```python
from build123d import *

# Parameters (mm, degrees)
BOSS_EXTRUDE1_DEPTH = 609.6
CUT_EXTRUDE1_DEPTH  = 38.1


with BuildPart() as part:
    # Sketch1 → Boss-Extrude1 (new body)
    with BuildSketch(Plane(origin=(0, 0, 0), x_dir=(1, 0, 0), z_dir=(0, 1, 0))):
        Polygon((13.746380944, 0), (9.720159182, 9.720159182), (0, 13.746380944), (-9.720159182, 9.720159182), (-13.746380944, 0), (-9.720159182, -9.720159182), (0, -13.746380944), (9.720159182, -9.720159182), align=None)
    extrude(amount=BOSS_EXTRUDE1_DEPTH)

    # Sketch2 → Cut-Extrude1 (cut)
    with BuildSketch(Plane(origin=(0, 609.6, 0), x_dir=(1, 0, 0), z_dir=(0, 1, 0))):
        Polygon((-1.00655544, -14.163309858), (-10.726714622, 9.303230267), (1.00655544, 14.163309858), (10.726714622, -9.303230267), align=None)
    extrude(amount=-CUT_EXTRUDE1_DEPTH, mode=Mode.SUBTRACT)


solid = part.part
```
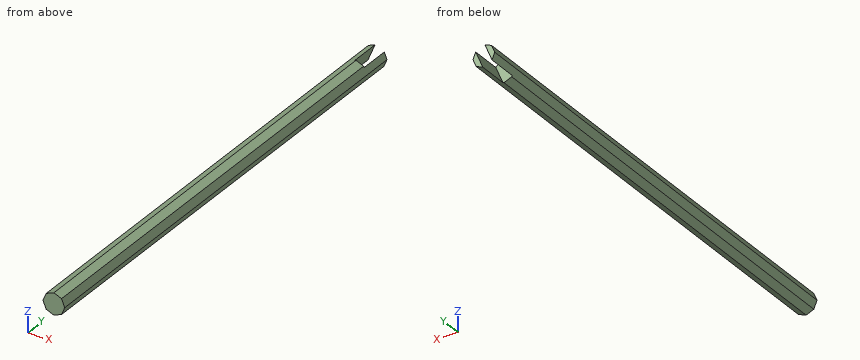
Read the model definition and answer for the solid it produces. Units are mm, in the model's axes. Give positions to 0.01 mm unless a question says otherwise; leave off trailing zeros. Write each loop counter-clockwise with the first axis right and the second up, starting at its lowest first coordinate (ties: lowest second). Pieces come first, ordered by that corner, then holes. Notation, with made-up numbers: (83, 79.25) - (91, 79.25) arc R9 cw to (91, 92.25) - close; hole circle Ø6 at (84.5, -12.75). An arc over 180 degrees is marked (long way). Write item = value, one per line. Start each with the question number.
Item 1: Each of these flat-tipped pins is pushed along its axis until it touches: P1, Ø4, axis at x = 7.5, y = 325.5, coming from the +Z side; P2, Ø1.5, axis at y = 313, z = -2, coming from the -X side; P3, Ø4, axis at y = 378.5, z = 7, coming from the +X side. Where does it stop, or does it pass through?
Item 2: Find the intervals of material crossed by probe 1 along X at (y, z) = (34.5, 9.5); probe 2 along Y at (x, z) = (4, 12); probe 3 along Z at (x, y) = (8.25, 161), in increasing order. Write a range as [from, to].
Item 3: Find section A-A (y = 50). Give the vertices of the cut face in (x, z).
Response:
q1.P1 = 11.47
q1.P2 = -13.23
q1.P3 = 11.68
q2.probe_1 = [-9.81, 9.81]
q2.probe_2 = [0, 571.5]
q2.probe_3 = [-10.33, 10.33]
q3.outline = (-13.75, 0) - (-9.72, -9.72) - (0, -13.75) - (9.72, -9.72) - (13.75, 0) - (9.72, 9.72) - (0, 13.75) - (-9.72, 9.72) - close
